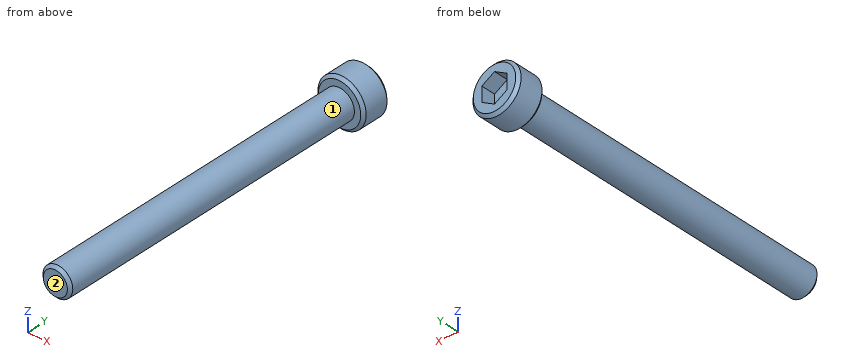
```python
from build123d import *

# Parameters (mm, degrees)
SKETCH1_W           = 3.3655
SKETCH1_H           = 4.064
SKETCH2_R           = 2.0828
BOSS_EXTRUDE1_DEPTH = 44.45
CUT_EXTRUDE1_DEPTH  = 2
CHAMFER1_SIZE       = 0.4


with BuildPart() as part:
    # Sketch1 → Revolve1 (revolve)
    with BuildSketch(Plane.XY, mode=Mode.PRIVATE) as revolve1_sk:
        with Locations((1.68275, 2.032)):
            Rectangle(SKETCH1_W, SKETCH1_H)
    revolve(revolve1_sk.sketch.rotate(Axis((0, 4.064, 0), (0, -1, 0)), 270), axis=Axis((0, 4.064, 0), (0, -1, 0)))

    # Sketch2 → Boss-Extrude1 (add)
    with BuildSketch(Plane.XZ):
        with Locations(Location((0, 0, 0), (0, 0, 270))):
            Circle(SKETCH2_R)
    extrude(amount=BOSS_EXTRUDE1_DEPTH)

    # Sketch3 → Cut-Extrude1 (cut)
    with BuildSketch(Plane(origin=(0, 4.064, 0), x_dir=(-1, 0, 0), z_dir=(0, 1, 0))):
        Polygon((-1.778, -1.026528779), (0, -2.053057557), (1.778, -1.026528779), (1.778, 1.026528779), (0, 2.053057557), (-1.778, 1.026528779), align=None)
    extrude(amount=-CUT_EXTRUDE1_DEPTH, mode=Mode.SUBTRACT)

    # Chamfer1
    chamfer1_edges = [part.edges().sort_by_distance(p)[0] for p in [
        (0, 0, 3.3655),
        (0, 4.064, 3.3655),
        (0, -44.45, 2.0828),
    ]]
    chamfer(chamfer1_edges, length=CHAMFER1_SIZE)


solid = part.part
```
Source: CAD feature listing. Evaluate the final solid. Frame: model axes, mm. Face numbers are marked on the shaded views. Give positions to 0.01 mm unless a question says otherwise; leave off trailing zeros. Loops run counter-clockwise (first coordinate to the right, second up) from the corner with the lowest first, then second, coordinate; pieces in that order, holes last. Notation, with made-up numbers: (49, 53) -> (66, 53) arc R30 ccw to (66, 77) -> close; hole circle Ø6 at (40.25, 19.25). An arc over 180 degrees is marked (long way). Use a Markdown table: item, result. Add a question column.
(1) First-contact query: pin 1 Ø1.8 at (x, z) = (0.5, -0.5) entering from +Y; pin 2 Ø2 at (x, z) = (-1.5, 1) entering from -Y; pin 3 Ø1.5 at (x, y) = (0.5, -33.5) entering from +Z; pin 4 Ø1.5 at (y, z) = (-4, -1) entering from +X. Flat tips, straight axial feed; report the tip coordinate or a pass-through.
(2) Section query B-B (y = -27). Output: boundary loops of the cut face in (x, z).
(3) Section query A-A (z = 0). Output: boundary loops of the cut face in (x, y).
(4) Pull-direction query (Y, two-part tool) for the marked faces 1 and 2; classes: +Y half, -Y half, draft (parallel to the pull), parting line (faces both ways), or undercut.
(5) Ray query, line 1 (Y direction, x = -0.25, z = 2.75); line 2 (Y direction, x = 0.25, z = -1.25); line 3 (Z direction, x = -1, y = -41). Return the intervals inside material, ascending.
Checked values:
| question | item | result |
|---|---|---|
| 1 | pin 1 | y = 2.06 |
| 1 | pin 2 | y = -44.45 |
| 1 | pin 3 | z = 2.08 |
| 1 | pin 4 | x = 2.07 |
| 2 | outline | circle Ø4.17 at (0, 0) |
| 3 | outline | (-3.37, 0.4) -> (-2.97, 0) -> (-2.08, 0) -> (-2.08, -44.05) -> (-1.68, -44.45) -> (1.68, -44.45) -> (2.08, -44.05) -> (2.08, 0) -> (2.97, 0) -> (3.37, 0.4) -> (3.37, 3.66) -> (2.97, 4.06) -> (1.78, 4.06) -> (1.78, 2.06) -> (-1.78, 2.06) -> (-1.78, 4.06) -> (-2.97, 4.06) -> (-3.37, 3.66) -> close |
| 4 | face 1 | draft |
| 4 | face 2 | -Y half |
| 5 | line 1 | 0 to 4.06 |
| 5 | line 2 | -44.45 to 2.06 |
| 5 | line 3 | -1.83 to 1.83 |
